from build123d import *

# Parameters (mm, degrees)
F0_W     = 63.5
F0_H     = 6.35
F1_DEPTH = 44.45
F2_SIZE  = 38.1
F3_SIZE  = 38.1
F4_R     = 4.2729711543
F4_R_2   = 4.6114221179
F4_R_3   = 3.96875
F5_DEPTH = 127
F6_R     = 6.35
F7_DEPTH = 127


with BuildPart() as f1:
    # F0 (on Front) → F1 (new body, symmetric)
    with BuildSketch(Plane.XZ):
        Polygon((1.8653165565, 15.875), (-4.4846834435, 15.875), (-4.4846834435, -15.875), (1.8653165565, -15.875), (1.8653165565, -9.525), align=None)
        with Locations((33.6153165565, -12.7)):
            Rectangle(F0_W, F0_H)
    extrude(amount=F1_DEPTH, both=True)

    # F2
    f2_edges = [f1.edges().sort_by_distance(p)[0] for p in [
        (65.365317, 44.45, -12.7),
    ]]
    chamfer(f2_edges, length=F2_SIZE)

    # F3
    f3_edges = [f1.edges().sort_by_distance(p)[0] for p in [
        (65.365317, -44.45, -12.7),
    ]]
    chamfer(f3_edges, length=F3_SIZE)

    # F4 (on Right) → F5 (cut, symmetric)
    with BuildSketch(Plane.YZ):
        Circle(F4_R)
        with Locations((19.05, 0)):
            Circle(F4_R_2)
        with Locations((-19.05, 0)):
            Circle(F4_R_3)
    extrude(amount=F5_DEPTH, both=True, mode=Mode.SUBTRACT)

    # F6 (on Top) → F7 (cut, symmetric)
    with BuildSketch(Plane.XY):
        with Locations((46.3153165565, 0)):
            Circle(F6_R)
    extrude(amount=F7_DEPTH, both=True, mode=Mode.SUBTRACT)


solid = f1.part
Model file for the job. Use its own axes, mm. A direction names the side the tool comes from. Coordinates: 2 decimals unless noted, no trailing zeros. Order: outer loops, then holes, each group sorted by start corner. A loop starts at its lowest first (then second) coordinate and runs counter-clockwise, first axis right, second up. Notation, with made-up numbers: M 58.5,-24 L 115.5,-24 A15 ccw 115.5,-15 Z; hole C 24,53 d6. An arc over 180 degrees is marked long. Return JSON: item names as keys, results as strings.
1. Tool access for faces 4 (the face through (26, -1, -9.525)), 5 (the face through (46.049, -25.667, -12.744)): list every direction of +Z, -Z, +X, -X, +Y, -Y with a clear straight run to the whole face (end or side of a thin tool).
Ans:
{"face 4": "+Z, +X, +Y, -Y", "face 5": "+Z, -Z, +X, -Y"}
2. Pull direction Y, two halves, no side cores. Call faces 1 (the face through (-1, -1, 15.875)), 2 (the face through (39.97, 0.28, -12.66)), 3 (the face through (46.049, 25.667, -12.744)): +Y half, -Y half, draft (parallel to the pull), parting line (faces both ways), or undercut.
Ans:
{"face 1": "draft", "face 2": "undercut", "face 3": "+Y half"}
3. Saw through at C-C (z = -11). Give the cut face in (x, y).
Ans:
{"outline": "M -4.48,-44.45 L 27.27,-44.45 L 65.37,-6.35 L 65.37,6.35 L 27.27,44.45 L -4.48,44.45 Z; hole C 46.32,0 d12.7"}
4. Saw through at B-B (z = 0). Give the cut face in (x, y), and give its area (3 significant figures).
Ans:
{"outline": "M -4.48,-44.45 L 1.87,-44.45 L 1.87,-23.02 L -4.48,-23.02 Z; M -4.48,-15.08 L 1.87,-15.08 L 1.87,-4.27 L -4.48,-4.27 Z; M -4.48,4.27 L 1.87,4.27 L 1.87,14.44 L -4.48,14.44 Z; M -4.48,23.66 L 1.87,23.66 L 1.87,44.45 L -4.48,44.45 Z", "area": "401 mm^2"}
5. Saw through at A-A (y = 19.05). Give the cut face in (x, z) (3 decimals), and give its area (3 significant figures).
Ans:
{"outline": "M -4.485,-15.875 L 52.665,-15.875 L 52.665,-9.525 L 1.865,-9.525 L 1.865,-4.611 L -4.485,-4.611 Z; M -4.485,4.611 L 1.865,4.611 L 1.865,15.875 L -4.485,15.875 Z", "area": "466 mm^2"}
6. Drill centre lines: probe 1 along Z at (x, y) = (0.6, 19.05) (3 decimals); probe 2 along Z at (x, y) = (-2, 0) (3 decimals); probe 3 along Z at (x, y) = (13.5, -10) (3 decimals). Where is each one in solid material? Low to high.
Ans:
{"probe 1": "-15.875 to -4.611, 4.611 to 15.875", "probe 2": "-15.875 to -4.273, 4.273 to 15.875", "probe 3": "-15.875 to -9.525"}
7. Saw through at D-D (x = 41.5). Give the cut face in (y, z) (3 decimals), and give its area (3 significant figures).
Ans:
{"outline": "M -30.215,-15.875 L -4.139,-15.875 L -4.139,-9.525 L -30.215,-9.525 Z; M 4.139,-15.875 L 30.215,-15.875 L 30.215,-9.525 L 4.139,-9.525 Z", "area": "331 mm^2"}
8. Flat gauge pins, fed straight in: pin 1 (9 mm diameter, centred on y = -19.05, z = 0, fed in from +X); pin 2 (6 mm diameter, centred on y = 22.5, z = -8, fed in from +X); pin 3 (19 mm diameter, centred on x = 26.5, y = -5, fed in from +Z) (3 decimals); pin 4 (5 mm diameter, centred on y = 0, z = 0, fed in from -X). Where does each tip first touch, or does it go through?
Ans:
{"pin 1": "x = 1.87", "pin 2": "x = 51.8", "pin 3": "z = -9.525", "pin 4": "through"}
